Study the drawing (mm; zero at the part's minimum x, y, z) and answer. Give positions to 0.01 mm unless a question says otherwise; leave off trailing zeros. Loops run counter-clockwise (first coordinate to the right, second up) from the corner with the lowest first, then second, coordinate; pieces in that order, holes last. Notation, with made-up numbers: (67.5, 1.5) - (126.5, 1.5) arc R31 cw to (126.5, 37.5) - close; hole circle Ø3 at (-35.75, 0.25). An arc over 180 degrees is marked (long way). Answer in a Markdown table with one row per item. Add a question column.
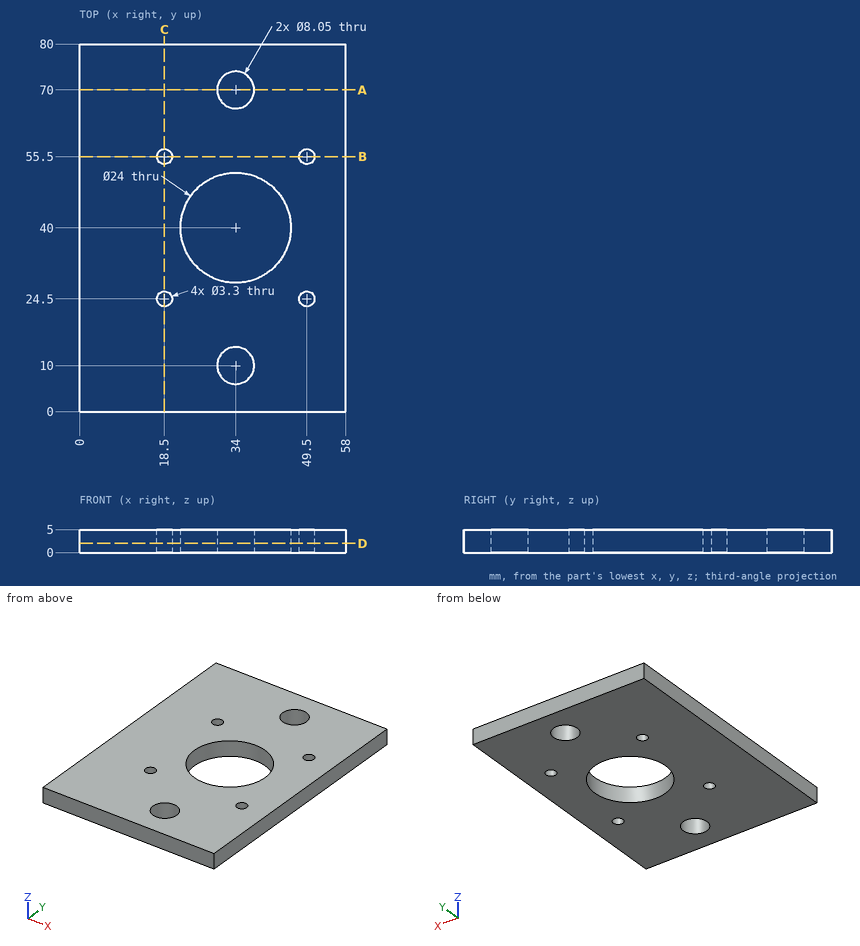
(1) A cutting plane is placed at C-C on x = 18.5. Determine the outline of the cut face in (y, z), plus the area to 3 significant figures.
(2) Given pin 1 Ø5 at (x, y) = (34, 10) entering from -Z, flat-ended and moving along its own axis, determine where the tip first touches the part or whether it passes through.
(3) Find the intervals of material crossed by line 1 along Y through (x, z) = (49.5, 2.6); line 2 along Y through (x, z) = (34, 1.4) (3 decimals); line 3 along X through (y, z) = (24, 4.35), in increasing order. Write a range as [from, to].
(4) A cutting plane is placed at A-A on y = 70. Determine the outline of the cut face in (x, z) (3 decimals), plus the area to 3 significant figures.
(5) A cutting plane is placed at B-B on y = 55.5. Determine the outline of the cut face in (x, z), plus the area to 3 significant figures.
(6) A cutting plane is placed at D-D on z = 2. Determine the outline of the cut face in (x, y) (3 decimals), plus the area to 3 significant figures.
Evaluation:
| question | item | result |
|---|---|---|
| 1 | outline | (0, 0) - (22.85, 0) - (22.85, 5) - (0, 5) - close; (26.15, 0) - (53.85, 0) - (53.85, 5) - (26.15, 5) - close; (57.15, 0) - (80, 0) - (80, 5) - (57.15, 5) - close |
| 1 | area | 367 mm² |
| 2 | pin 1 | passes through |
| 3 | line 1 | y = [0, 22.85], [26.15, 53.85], [57.15, 80] |
| 3 | line 2 | y = [0, 5.975], [14.025, 28], [52, 65.975], [74.025, 80] |
| 3 | line 3 | x = [0, 16.93], [20.07, 47.93], [51.07, 58] |
| 4 | outline | (0, 0) - (29.975, 0) - (29.975, 5) - (0, 5) - close; (38.025, 0) - (58, 0) - (58, 5) - (38.025, 5) - close |
| 4 | area | 250 mm² |
| 5 | outline | (0, 0) - (16.85, 0) - (16.85, 5) - (0, 5) - close; (20.15, 0) - (47.85, 0) - (47.85, 5) - (20.15, 5) - close; (51.15, 0) - (58, 0) - (58, 5) - (51.15, 5) - close |
| 5 | area | 257 mm² |
| 6 | outline | (0, 0) - (58, 0) - (58, 80) - (0, 80) - close; hole circle Ø3.3 at (18.5, 24.5); hole circle Ø3.3 at (18.5, 55.5); hole circle Ø24 at (34, 40); hole circle Ø8.05 at (34, 10); hole circle Ø8.05 at (34, 70); hole circle Ø3.3 at (49.5, 24.5); hole circle Ø3.3 at (49.5, 55.5) |
| 6 | area | 4,050 mm² |
